Input: dimensioned drawing with shaded views. Units: mm. Origin: part minimum x, y, z. A direction names the side the tool comes from. Give positions to 0.01 mm unless a question says otherwise; leave off trailing zeros. Order: outer loops, then holes, each group sorted by start corner. A loop starts at its lowest first (then second) coordinate and runs counter-clockwise, first axis right, second up.
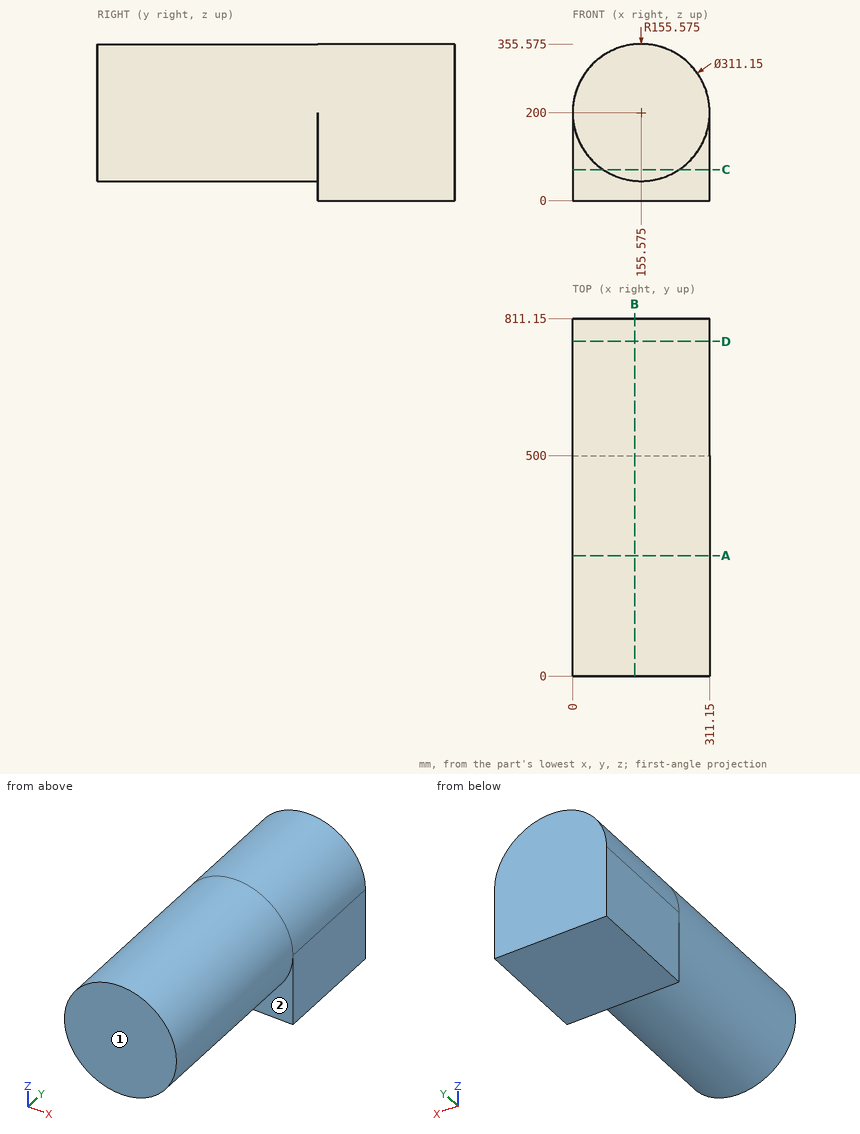
1) Pin query (flat end, axial travel): pin 1 (8 mm diameter, centred on x = 95.5, y = 229.5, fed in from -Z); pin 2 (3 mm diameter, centred on x = 191, y = 302.5, fed in from +Z); pin 3 (1 mm diameter, centred on x = 170, z = 37, fed in from -Y). Return the tip coordinate at first contact, or that it passes through.
Report:
pin 1: stops at z = 54.88
pin 2: stops at z = 351.83
pin 3: stops at y = 500
2) Material intervals for L1, parallel to X at y = 232.5, z = 205.5; L2, parallel to Z at x = 163.5, y = 244; L3, parallel to X at y = 369, z = 97, sorted ascending.
Report:
L1: x = 0.1 to 311.05
L2: z = 44.63 to 355.37
L3: x = 38.98 to 272.17
3) Section query B-B, the plane x = 140.5. Return the cut outline in (y, z).
Report:
outline: (0, 45.16) - (500, 45.16) - (500, 0) - (811.15, 0) - (811.15, 354.84) - (0, 354.84) - close
4) Reachability of the marked faces 1 and 2 from +Z, -Z, +X, -X, +Y, -Y: full face, straight path, thin tool, end or side. Return the list, or none.
Report:
face 1: +Z, -Z, +X, -X, -Y
face 2: -Z, -Y
5) Section query D-D, the plane y = 759.5. Return the cut outline in (x, z) (3 decimals).
Report:
outline: (0, 0) - (311.15, 0) - (311.15, 200) arc R155.575 ccw to (0, 200) - close
6) Section query A-A, the plane y = 273. Return the cut outline in (x, z) (3 decimals), and give its area (3 significant figures).
Report:
outline: circle Ø311.15 at (155.575, 200)
area: 76,000 mm2
7) Section query C-C, the plane z = 70.5. Return the cut outline in (x, y).
Report:
outline: (0, 500) - (69.36, 500) - (69.36, 0) - (241.79, 0) - (241.79, 500) - (311.15, 500) - (311.15, 811.15) - (0, 811.15) - close
